Part model, mm, in its own coordinate system. A direction names the side the tool comes from. Give positions to 0.01 mm unless a question says otherwise; leave off trailing zeros. Loops run counter-clockwise (first coordinate to the right, second up) from the corner with the lowest first, then second, coordinate; pieces in that order, holes last. Notation, with made-up numbers: (79, 27) -> (136, 27) arc R20 cw to (136, 46) -> close; hole circle Ø5 at (64.5, -6.5). An arc over 180 degrees is marked (long way). Write item = value, one per line.
from build123d import *

# Parameters (mm, degrees)
EXTRUDE1_DEPTH     = 40
CUT_EXTRUDE3_DEPTH = 2.42


with BuildPart() as part:
    # Sketch1 → Extrude1 (new body)
    with BuildSketch(Plane.XY):
        Polygon((0, 0), (0, -25.22), (25.22, -25.22), (25.22, -23.8), (1.42, -23.8), (1.42, 0), align=None)
    extrude(amount=EXTRUDE1_DEPTH)

    # Sketch3 → Cut-Extrude3 (cut, through all)
    with BuildSketch(Plane(origin=(0, -23.8, 0), x_dir=(-1, 0, 0), z_dir=(0, 1, 0))):
        Polygon((-1.42, 40), (-1.42, 16.2), (-2.84, 16.2), (-2.84, 19.4), (-10.8, 19.4), (-10.8, 22), (-17.85, 22), (-17.85, 19.4), (-25.22, 19.4), (-25.22, 40), align=None)
    extrude(amount=-CUT_EXTRUDE3_DEPTH, mode=Mode.SUBTRACT)


solid = part.part
1) Which spindle directions (+Z, -Z, +X, -X, +Y, -Y) get a long thin tool onto all of the face, cutting with end or side? Do faces 5 (the face through (1, -16, 0)), 6 (the face through (7, -25, 19.4)), 7 (the face through (14, -25, 22)), 8 (the face through (13, -23.8, 11)). Say none if no direction does.
Resolved:
face_5 = -Z, +X, -X, +Y, -Y
face_6 = +Z, +Y, -Y
face_7 = +Z, +X, +Y, -Y
face_8 = +Z, -Z, +X, +Y
2) Pull direction X, two halves, no side cores. Call faces 1 (the face through (17.85, -25, 21)), 2 (the face through (10.8, -25, 21)), 3 (the face through (0, -12, 20)), 4 (the face through (2.84, -25, 18)): pulls with the +X half, pulls with the -X half, needs draft (parallel to the pull), parting line crosses it, or undercut.
Resolved:
face_1 = pulls with the +X half
face_2 = undercut
face_3 = pulls with the -X half
face_4 = undercut
3) Slice it at C-C, the plane x = 7.5. List the corners of the cut face in (y, z).
Resolved:
outline = (-25.22, 0) -> (-23.8, 0) -> (-23.8, 19.4) -> (-25.22, 19.4) -> close
4) Drop flat-ended pins along their axis: P1, Ø1, axis at y = -21.5, z = 35, coming from the -X side; P2, Ø7.5, axis at y = -10, z = 13.5, coming from the +X side; P3, Ø2, axis at x = 8, y = -22, coming from the -Z side; P4, Ø6.5, axis at x = 10, z = 8.5, coming from the +Y side. Give the stop position or say it passes through.
Resolved:
P1 = 0
P2 = 1.42
P3 = through
P4 = -23.8
5) Drill centre lines: line 1 along X through (y, z) = (-16, 13); line 2 along Y through (x, z) = (22.5, 7.5). Where is each one in solid material? Low to high. Write a range as [from, to].
Resolved:
line_1 = [0, 1.42]
line_2 = [-25.22, -23.8]
6) Slice it at A-A, the plane z = 12.5. List the corners of the cut face in (x, y).
Resolved:
outline = (0, -25.22) -> (25.22, -25.22) -> (25.22, -23.8) -> (1.42, -23.8) -> (1.42, 0) -> (0, 0) -> close
7) Slice it at B-B, the plane y = -6.5. List the corners of the cut face in (x, z), and give its area (3 significant figures).
Resolved:
outline = (0, 0) -> (1.42, 0) -> (1.42, 40) -> (0, 40) -> close
area = 56.8 mm²
